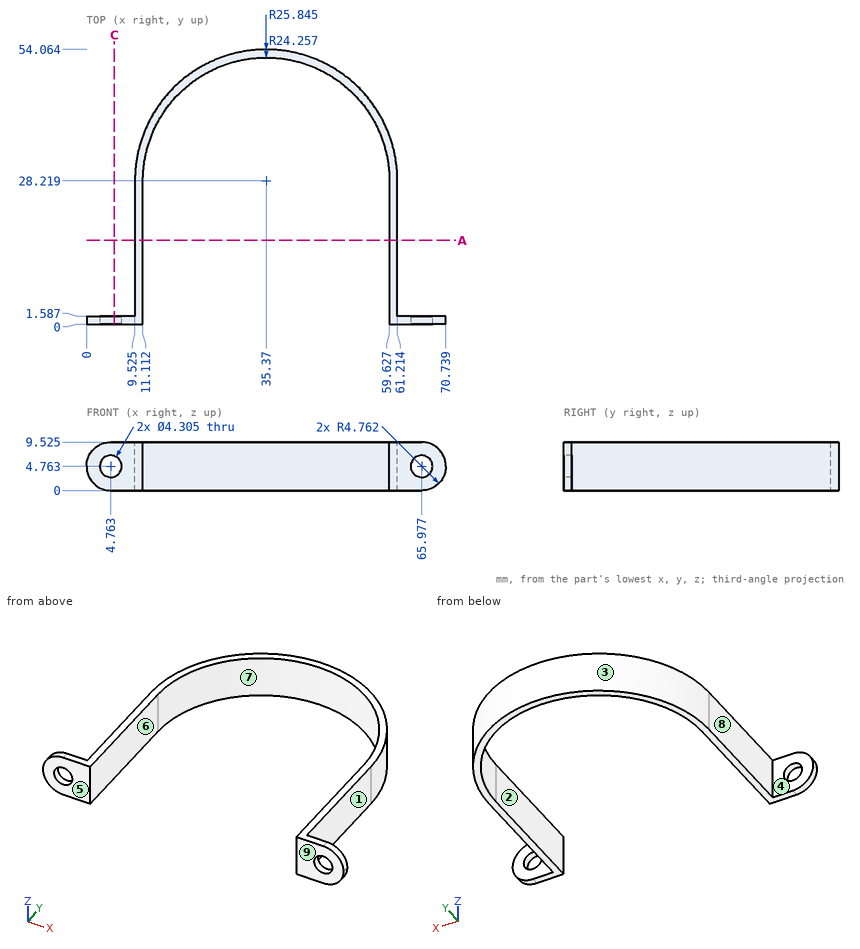
The drawing under review shows one solid part. Ordinate dimensions are in mm from its lowest x, y, z. A direction names the side the tool comes from. Round coordinates to 2 decimals unless told otherwise and drop trailing zeros. Loops run counter-clockwise (first coordinate to the right, second up) from the corner with the lowest first, then second, coordinate; pieces in that order, holes last. Notation, with made-up numbers: (67.5, -21.5) - (113.5, -21.5) arc R31 ccw to (113.5, 6.5) - close; hole circle Ø6 at (29, 51). An arc over 180 degrees is marked (long way). One line per item, written item: value. Start each with the question number.
1) Insertion check: pin 1 Ø3 at (y, z) = (12, 6.5) entering from +X; pin 2 Ø5 at (x, z) = (67, 2.5) entering from +Y; pin 3 Ø4 at (y, z) = (22.5, 7) entering from -X (1 decimal). Each pin has a flat end and moves straight along its axis. Give the tip position at first contact, or say it passes through.
2) Draft analysis for pull direction X (two halves, no side actions). For the marked faces 6, 7, 8 and 9, state which applies: +X half, -X half, draft (parallel to the pull), parting line (faces both ways), or undercut.
3) Consider section C-C on x = 5.5. Give the boundary of the cut face in (y, z) (1 decimal).
4) To check wall thickness, follow L1, parallel to X at y = 27, z = 1.75 (1 decimal); L2, parallel to Y at x = 7, z = 2.25; L3, parallel to X at y = 39, z = 8.5. State the ranges of each line that lie inside material, in increasing order. Write a range as from..to.
5) Consider section A-A on y = 16.5. Give the boundary of the cut face in (x, z) (1 decimal).
6) For the marked faces 1, 2, 3, 4 and 5, list the 3-axis set-ups (+Z, -Z, +X, -X, +Y, -Y) from which the entire face can be reached by the end or side of a thin tool; tool diameter is ignored.
Reported:
1. pin 1: stops at x = 61.21
1. pin 2: stops at y = 1.59
1. pin 3: stops at x = 9.5
2. face 6: undercut
2. face 7: undercut
2. face 8: -X half
2. face 9: draft
3. outline: (0, 0) - (1.6, 0) - (1.6, 2.7) - (0, 2.7) - close; (0, 6.8) - (1.6, 6.8) - (1.6, 9.5) - (0, 9.5) - close
4. L1: x = 9.5..11.1, 59.6..61.2
4. L2: y = 0..1.59
4. L3: x = 11.88..13.64, 57.1..58.86
5. outline: (9.5, 0) - (11.1, 0) - (11.1, 9.5) - (9.5, 9.5) - close; (59.6, 0) - (61.2, 0) - (61.2, 9.5) - (59.6, 9.5) - close
6. face 1: +Z, -Z, +X, +Y
6. face 2: +Z, -Z, -Y
6. face 3: +Z, -Z, +Y
6. face 4: +Z, -Z, -X, +Y
6. face 5: +Z, -Z, +X, -X, -Y
